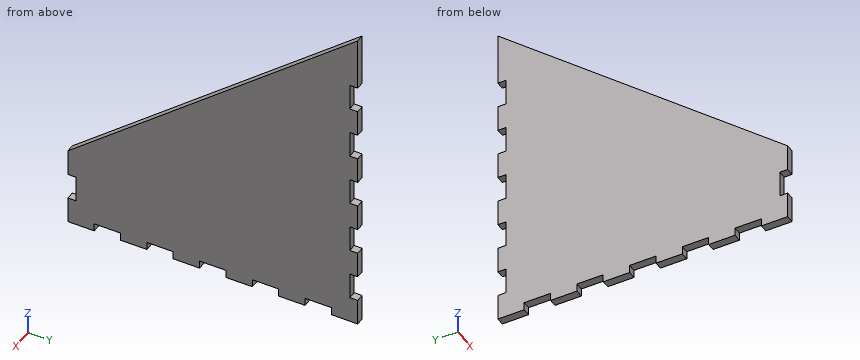
```python
from build123d import *

# Parameters (mm, degrees)
F1_DEPTH = 3
F2_W     = 10
F2_H     = 3
F3_DEPTH = 25
F4_W     = 3
F4_H     = 10
F5_DEPTH = 25
F6_W     = 3
F6_H     = 10
F7_DEPTH = 25


with BuildPart() as f1:
    # F0 (on Right) → F1 (new body)
    with BuildSketch(Plane.YZ):
        Polygon((0, 0), (110, 0), (110, 120), (0, 30), align=None)
    extrude(amount=F1_DEPTH)

    # F2 (on face) → F3 (cut)
    with BuildSketch(Plane.YZ.offset(3)):
        with Locations((15, 1.5)):
            Rectangle(F2_W, F2_H)
        with Locations((35, 1.5)):
            Rectangle(F2_W, F2_H)
        with Locations((55, 1.5)):
            Rectangle(F2_W, F2_H)
        with Locations((75, 1.5)):
            Rectangle(F2_W, F2_H)
        with Locations((95, 1.5)):
            Rectangle(F2_W, F2_H)
    extrude(amount=-F3_DEPTH, mode=Mode.SUBTRACT)

    # F4 (on face) → F5 (cut)
    with BuildSketch(Plane.YZ.offset(3)):
        with Locations((1.5, 15)):
            Rectangle(F4_W, F4_H)
    extrude(amount=-F5_DEPTH, mode=Mode.SUBTRACT)

    # F6 (on face) → F7 (cut)
    with BuildSketch(Plane.YZ.offset(3)):
        with Locations((108.5, 15)):
            Rectangle(F6_W, F6_H)
        with Locations((108.5, 35)):
            Rectangle(F6_W, F6_H)
        with Locations((108.5, 55)):
            Rectangle(F6_W, F6_H)
        with Locations((108.5, 75)):
            Rectangle(F6_W, F6_H)
        with Locations((108.5, 95)):
            Rectangle(F6_W, F6_H)
    extrude(amount=-F7_DEPTH, mode=Mode.SUBTRACT)


solid = f1.part
```
Read the model definition and answer for the solid it produces. Units are mm, in the model's axes. Coordinates: 2 decimals unless noted, no trailing zeros. Order: outer loops, then holes, each group sorted by start corner. A loop starts at its lowest first (then second) coordinate and runs counter-clockwise, first axis right, second up. Notation, with made-up numbers: (8.25, -38) - (34.25, -38) arc R14 cw to (34.25, -23) - close; hole circle Ø6 at (-34.75, -37.5). An arc over 180 degrees is marked (long way). Answer as a JSON object with one key per item and string values. Group by question number.
Item 1: Section B-B (y = 77) is taken. Give the vertices of the cut face in (x, z).
Item 2: Section A-A (z = 75) is taken. Give the vertices of the cut face in (x, y), plus the area to 3 significant figures.
Item 3: Consider probe 1 along Y at (x, z) = (0.9, 15); probe 2 along Z at (x, y) = (1.45, 58); probe 3 along Y at (x, z) = (2.1, 53.5). Determine where each line is inside the solid, lowest interval first. Write a range as from..to.
Item 4: Flat-ended cylindrical pins translate along their axes: P1, Ø1.5, axis at x = 2, y = 17, coming from the -Z side; P2, Ø0.9, axis at x = 1, y = 108, coming from the +Z side; P3, Ø1.5, axis at x = 1, y = 82, coming from the +Z side. Find the tip coordinate at first contact, or state that the pin passes through.
Results are:
{
 "1": {"outline": "(0, 3) - (3, 3) - (3, 93) - (0, 93) - close"},
 "2": {"outline": "(0, 55) - (3, 55) - (3, 107) - (0, 107) - close", "area": "156 mm^2"},
 "3": {"probe 1": "y = 3..107", "probe 2": "z = 3..77.45", "probe 3": "y = 28.72..107"},
 "4": {"P1": "stops at z = 3", "P2": "stops at z = 118.73", "P3": "stops at z = 97.7"}
}
